from build123d import *

# Parameters (mm, degrees)
BOSS_EXTRUDE1_DEPTH     = 2.54
SKETCH3_R               = 1.5000000000000009
BOSS_EXTRUDE2_DEPTH     = 1.5875
FILLET1_START           = -12.7000001
FILLET1_DEPTH           = 25.4000001
FILLET1_START_2         = -5
FILLET1_2_DEPTH         = 10
FILLET2_R               = 2.54
SKETCH4_R               = 3.5
BOSS_EXTRUDE3_DEPTH     = 7
SKETCH5_R               = 1.75
CUT_EXTRUDE1_DEPTH      = 45.14049388033623
CUT_EXTRUDE2_DEPTH      = 39.723935750385714
CUT_EXTRUDE2_DEPTH_BACK = 2
SKETCH6_R               = 3.5
SKETCH10_R              = 4.77
SKETCH10_R_2            = 3.5
BOSS_EXTRUDE4_DEPTH     = 21.844000000000005
SKETCH9_R               = 1.7499999999999998
CUT_EXTRUDE4_DEPTH      = 43.12113483751359
CUT_EXTRUDE5_DEPTH      = 45.62315381335121
CUT_EXTRUDE5_DEPTH_BACK = 45.62315381335121


with BuildPart() as part:
    # Sketch1 → Boss-Extrude1 (new body)
    with BuildSketch(Plane(origin=(0, 0, 0), x_dir=(1, 0, 0), z_dir=(0, 1, 0))):
        Polygon((-12.7, 12.699999999999998), (12.7, 12.699999999999998), (12.700000000000003, -12.700000000000001), (-12.699999999999996, -12.700000000000001), align=None)
    extrude(amount=BOSS_EXTRUDE1_DEPTH)

    # Sketch3 → Boss-Extrude2 (add, symmetric)
    with BuildSketch(Plane(origin=(0, 0, 0), x_dir=(0, 0, -1), z_dir=(1, 0, 0))):
        with BuildLine():
            Line((-22.53488, 28.691839999999996), (-14.109077453558108, 14.51812311143032))
            ThreePointArc((-14.109077453558108, 14.51812311143032), (-12.3014463794853, 9.646212675108597), (-12.336895325054973, 4.449888515498061))
            Line((-12.336895325054973, 4.449888515498061), (-12.700000000000001, 2.54))
            Line((-12.700000000000001, 2.54), (12.699999999999998, 2.54))
            Line((12.699999999999998, 2.54), (-13.91324894993197, 33.77463750916512))
            ThreePointArc((-13.91324894993197, 33.77463750916512), (-20.3599032710008, 34.856128324475804), (-22.53488, 28.691839999999996))
        make_face()
        with Locations((-17.779999999999998, 30.479999999999997)):
            Circle(SKETCH3_R, mode=Mode.SUBTRACT)
    extrude(amount=BOSS_EXTRUDE2_DEPTH, both=True)

    # Fillet1: read off the stored shape, not the designer's step
    # Fillet1 outline → Fillet1 (add)
    with BuildSketch(Plane.XY.offset(FILLET1_START)):
        with BuildLine():
            ThreePointArc((-1.5875, 5.08), (-2.331448776, 3.283948776), (-4.1275, 2.54))
            Line((-4.1275, 2.54), (-1.5875, 2.54))
            Line((-1.5875, 2.54), (-1.5875, 5.08))
        make_face()
        with BuildLine():
            Line((1.5875, 2.54), (4.1275, 2.54))
            ThreePointArc((4.1275, 2.54), (2.331448776, 3.283948776), (1.5875, 5.08))
            Line((1.5875, 5.08), (1.5875, 2.54))
        make_face()
    extrude(amount=FILLET1_DEPTH)

    # Fillet1 2 outline → Fillet1 2 (cut)
    with BuildSketch(Plane.YZ.offset(FILLET1_START_2)):
        Polygon((5.08, -10.535811211), (2.54, -12.7), (5.08, -12.7000001), align=None)
        with BuildLine():
            Line((5.08, 12.7), (2.54, 12.7))
            Line((2.54, 12.7), (4.449888515, 12.336895325))
            ThreePointArc((4.449888515, 12.336895325), (4.764360857, 12.280707955), (5.08, 12.231496116))
            Line((5.08, 12.231496116), (5.08, 12.7))
        make_face()
    extrude(amount=FILLET1_2_DEPTH, mode=Mode.SUBTRACT)

    # Fillet2
    fillet2_edges = [part.edges().sort_by_distance(p)[0] for p in [
        (12.7, 1.27, -12.699999999999998),
        (12.700000000000003, 1.27, 12.700000000000001),
        (-12.699999999999996, 1.27, 12.700000000000001),
        (-12.7, 1.27, -12.699999999999998),
    ]]
    fillet(fillet2_edges, radius=FILLET2_R)

    # Sketch4 → Boss-Extrude3 (add)
    with BuildSketch(Plane.XZ):
        Circle(SKETCH4_R)
    extrude(amount=-BOSS_EXTRUDE3_DEPTH)

    # Sketch5 → Cut-Extrude1 (cut, through all)
    with BuildSketch(Plane.XZ):
        with Locations(Location((0, 0, 0), (0, 0, 270))):
            Circle(SKETCH5_R)
    extrude(amount=-CUT_EXTRUDE1_DEPTH, mode=Mode.SUBTRACT)

    # Sketch6 → Cut-Extrude2 (cut, two sides: drawn at the far end of the back side and taken through both)
    with BuildSketch(Plane(origin=(0, 7, 0), x_dir=(1, 0, 0), z_dir=(0, 1, 0)).offset(-CUT_EXTRUDE2_DEPTH_BACK)):
        Circle(SKETCH6_R)
    extrude(amount=CUT_EXTRUDE2_DEPTH + CUT_EXTRUDE2_DEPTH_BACK, mode=Mode.SUBTRACT)

    # Sketch10 → Boss-Extrude4 (add)
    with BuildSketch(Plane(origin=(0, 2.54, 0), x_dir=(1, 0, 0), z_dir=(0, 1, 0))):
        with Locations(Location((0, 0, 0), (0, 0, 70.560627051))):
            Circle(SKETCH10_R)
        with Locations(Location((0, 0, 0), (0, 0, 270))):
            Circle(SKETCH10_R_2, mode=Mode.SUBTRACT)
    extrude(amount=BOSS_EXTRUDE4_DEPTH)

    # Sketch9 → Cut-Extrude4 (cut, through all)
    with BuildSketch(Plane(origin=(0, 2.54, 0), x_dir=(1, 0, 0), z_dir=(0, 1, 0))):
        with Locations(Location((-9.524999999999999, -9.525000000000002, 0), (0, 0, 270))):
            Circle(SKETCH9_R)
        with Locations(Location((-9.524999999999999, 9.524999999999999, 0), (0, 0, 270))):
            Circle(SKETCH9_R)
        with Locations(Location((9.525000000000002, 9.525000000000002, 0), (0, 0, 270))):
            Circle(SKETCH9_R)
        with Locations(Location((9.525000000000002, -9.524999999999999, 0), (0, 0, 270))):
            Circle(SKETCH9_R)
    extrude(amount=-CUT_EXTRUDE4_DEPTH, mode=Mode.SUBTRACT)

    # Sketch8 → Cut-Extrude5 (cut, two sides: drawn at the far end of the back side and taken through both)
    with BuildSketch(Plane(origin=(1.5875, 0, 0), x_dir=(0, 0, -1), z_dir=(1, 0, 0)).offset(-CUT_EXTRUDE5_DEPTH_BACK)):
        Polygon((-9.955433984779507, 29.129548290728966), (6.7091639016479245, 9.571144309395804), (6.709163901647932, 29.129548290728973), align=None)
    extrude(amount=CUT_EXTRUDE5_DEPTH + CUT_EXTRUDE5_DEPTH_BACK, mode=Mode.SUBTRACT)


solid = part.part
Design review of the part built by this model. Coordinates are the model's own, in mm. A direction names the side the tool comes from. Coordinates: 2 decimals unless noted, no trailing zeros. Order: outer loops, then holes, each group sorted by start corner. A loop starts at its lowest first (then second) coordinate and runs counter-clockwise, first axis right, second up. Notation, with made-up numbers: (76.5, 76.5) - (92.5, 76.5) arc R25 cw to (92.5, 91.5) - close; hole circle Ø10 at (49, 77). An arc over 180 degrees is marked (long way). Put each result on its own line as item: value.
1) Take a section at D-D, the plane y = 14. Give the boundary of the cut face in (x, z), and give its area (3 significant figures).
Response values:
outline: (-3.76, -2.94) - (-1.91, -2.94) arc R3.5 cw (long way) to (1.91, -2.94) - (3.76, -2.94) arc R4.77 ccw to (1.59, 4.5) - (1.59, 13.82) - (-1.59, 13.82) - (-1.59, 4.5) arc R4.77 ccw to start
area: 53.8 mm²
2) Wall thickness on L1, parallel to X at y = 10.25, z = 0; L2, parallel to Y at x = -5.75, z = -8; L3, parallel to X at y = 19, z = 16: over which ranges is each line inside the solid? List them lowest first. Write a range as from..to.
Response values:
L1: x = -4.77..-3.5, 3.5..4.77
L2: y = 0..2.54
L3: x = -1.59..1.59
3) Take a section at B-B, the plane z = 17.78. Give the boundary of the cut face in (x, y).
Response values:
outline: (-1.59, 20.69) - (1.59, 20.69) - (1.59, 28.98) - (-1.59, 28.98) - close; (-1.59, 31.98) - (1.59, 31.98) - (1.59, 35.56) - (-1.59, 35.56) - close
4) Take a section at C-C, the plane y = 30.48. Give the boundary of the cut face in (x, z).
Response values:
outline: (-1.59, 11.11) - (1.59, 11.11) - (1.59, 16.28) - (-1.59, 16.28) - close; (-1.59, 19.28) - (1.59, 19.28) - (1.59, 22.86) - (-1.59, 22.86) - close
5) Take a section at A-A, the plane x = 0. Give the boundary of the cut face in (y, z), and give its area (3 significant figures).
Response values:
outline: (0, -12.7) - (2.54, -12.7) - (13.34, -3.5) - (5, -3.5) - (5, -1.75) - (0, -1.75) - close; (0, 1.75) - (5, 1.75) - (5, 3.5) - (21.55, 3.5) - (33.77, 13.91) arc R5.08 ccw to (28.69, 22.53) - (14.52, 14.11) arc R14.43 cw to (4.45, 12.34) - (2.54, 12.7) - (0, 12.7) - close; hole circle Ø3 at (30.48, 17.78)
area: 469 mm²
6) Tool access review of faces 1 (the face through (0.27, 11.32, 3.49)), 2 (the face through (1.588, 21, 12)), 3 (the face through (-4.614, 10.248, 1.21)), 4 (the face through (-2.312, 3.304, -7.618)): name each direction out of +Z, -Z, +X, -X, +Y, -Y from which nothing blocks a thin tool from reaching the whole face with its end or side.
Response values:
face 1: +Y
face 2: +Z, +X, +Y
face 3: -X, +Y
face 4: -Z, -X, +Y
7) The part is to be moulded in two halves that separate along Z. For faces 5 (the face through (-11.08, 1.29, 10.33)), 6 (the face through (2.351, 3.264, -7.618)), 7 (the face through (0, 1, 12.7)), say which applies: released by +Z, released by -Z, zero draft, split by the parting line, or undercut.
Response values:
face 5: undercut
face 6: zero draft
face 7: released by +Z
8) Insertion check: P1, Ø6, axis at x = -0.5, z = 19, coming from the -Y side; P2, Ø14.5, axis at y = 14.5, z = 9.5, coming from the -X side; P3, Ø12, axis at y = 18, z = 13, coming from the +X side. Each pin has a flat end and moves straight along its axis. Give the tip position at first contact, or say it passes through.
Response values:
P1: stops at y = 17.7
P2: stops at x = -4.21
P3: stops at x = 1.59
